Build history of the part. All positions in model axes, mm. A direction names the side the tool comes from. Give positions to 0.01 mm unless a question says otherwise; leave off trailing zeros. Order: outer loops, then holes, each group sorted by start corner. A loop starts at its lowest first (then second) coordinate and runs counter-clockwise, first axis right, second up. Notation, with made-up numbers: (-21, 63) -> (-17, 63) arc R21 ccw to (-17, 71) -> close; hole circle Ø7 at (36, -19). An arc over 180 degrees is marked (long way). One line per question, with ' | ' between items. Start each with the question number.
(1) Drill centre lines: L1, parallel to Z at x = 0, y = 3.5; L2, parallel to Z at x = 0.9, y = 4.75; L3, parallel to Y at x = 0.05, z = -4.75. Where is each one in solid material? Low to high. Write a range as from..to.
(2) Cut at A-A (z = -5.5). Give the cut face in (x, y).
(3) Pin check, flat tip, straight feed: pin 1 Ø1.8 at (x, z) = (0, -5.5) entering from -Y. Stop position of the tip, or through.
(4) Which spindle directions (+Z, -Z, +X, -X, +Y, -Y) get a long thin tool onto all of the face, cutting with end or side? Do faces 4 (the face through (0.13, 2.96, -6.49)), 5 (the face through (0, 15, -7.5)). Say none if no direction does.
(5) Pull direction X, two halves, no side cores. Call faces 1 (the face through (-2, 15, 0)), 2 (the face through (0, 0, 0)), 3 (the face through (0.13, 2.96, 4.51)): +X half, -X half, draft (parallel to the pull), parting line (faces both ways), or undercut.
(6) Cut at B-B (x = 0). Give the cut face in (y, z).
Autodesk Inventor part; units mm, degrees
ref_plane "YZ Plane" through (0, 0, 0) normal (1, 0, 0) x (0, 1, 0)
ref_plane "XZ Plane" through (0, 0, 0) normal (0, 1, 0) x (-1, 0, 0)
ref_plane "XY Plane" through (0, 0, 0) normal (0, 0, 1) x (1, 0, 0)
sketch "スケッチ1" plane through (0, 0, 0) normal (0, 1, 0) x (-1, 0, 0)
  line L0 (-2, 7.5) -> (2, 7.5)
  line L1 (2, 7.5) -> (2, -7.5)
  line L2 (2, -7.5) -> (-2, -7.5)
  line L3 (-2, -7.5) -> (-2, 7.5)
  line L4 (-2, 7.5) -> (2, -7.5) construction
  line L5 (2, 7.5) -> (-2, -7.5) construction
  circle A0 centre (0, 5.5) radius 1
  circle A1 centre (0, -5.5) radius 1
  line L6 (0, 5.5) -> (0, 7.5) construction
  line L7 (0, -5.5) -> (0, -7.5) construction
  point P0 (0, 0)
  dimension "d0" = 4
  dimension "d1" = 15
  dimension "d2" = 2
  dimension "d3" = 2
extrude "押し出し1" add sketch "スケッチ1" along normal blind 30 contours L0 L1 L2 L3 | A0 | A1
extrude "押し出し2" cut sketch "スケッチ1" along normal blind 6 contours A0 | A1
properties part number "BallSensor_Mount"
Result set:
1) L1: z = -7.5..-6.5, -4.5..4.5, 6.5..7.5 | L2: z = -7.5..-5.94, -5.06..5.06, 5.94..7.5 | L3: y = 6..30
2) outline: (-2, 0) -> (-1, 0) -> (-1, 6) -> (1, 6) -> (1, 0) -> (2, 0) -> (2, 30) -> (-2, 30) -> close
3) pin 1: stops at y = 6
4) face 4: -Y | face 5: -Z, +X, -X, +Y, -Y
5) face 1: -X half | face 2: draft | face 3: undercut
6) outline: (0, -7.5) -> (30, -7.5) -> (30, 7.5) -> (0, 7.5) -> (0, 6.5) -> (6, 6.5) -> (6, 4.5) -> (0, 4.5) -> (0, -4.5) -> (6, -4.5) -> (6, -6.5) -> (0, -6.5) -> close
